The listing builds one solid part. Answer for the finished solid, in the listing's coordinates (mm). A direction names the side the tool comes from. Give positions to 0.01 mm unless a question says otherwise; leave off trailing zeros. Order: outer loops, then holes, each group sorted by start corner. A loop starts at its lowest first (then second) coordinate and runs counter-clockwise, first axis right, second up. Notation, with made-up numbers: (43, 26) - (60, 26) arc R16 ccw to (60, 30) - close; hole circle Ø2 at (85.25, -35). An arc over 180 degrees is marked (long way). Answer as CSV lines item,"result". Start each with the question number.
1. Section C-C on z = 1.9 is taken. Give the vertices of the cut face in (x, y), and give its area (3 significant figures).
2. Section B-B on y = -45 is taken. Give the vertices of the cut face in (x, z), and give its area (4 significant figures).
3. Section D-D on y = -35 is taken. Give the vertices of the cut face in (x, z), and give its area (3 significant figures).
4. Which of the six approach directions +Z, -Z, +X, -X, +Y, -Y give full straight-line access (tool end or side, diameter ignored) to faces 4 (the flat face through (4, -25, 1)), 5 (the flat face through (68, -32, 2.5))?
5. Section A-A on x = 119 is taken. Give the vertices of the cut face in (y, z).
6. A flat-ended cylindrical pin translates along its axis: pin 1 (1.2 mm diameter, centred on x = 132.5, z = 1, fed in from +Y). Find the tip coordinate at first contact, or state that the pin passes through.
7. Determine the mould class of faces 1 (the flat face through (68, -32, 0)), 2 (the flat face through (0, -33, 1)), 3 (the cylindrical face through (117.45, -34.93, 1.27)) for opening direction X: +X half, -X half, draft (parallel to the pull), parting line (faces both ways), or undercut.
8. Consider line 1 along Y through (x, z) = (119, 1.5); line 2 along X through (y, z) = (-6, 2.25); line 3 along X through (y, z) = (-21, 0.7). Determine where each line is inside the solid, lowest interval first. Write a range as [from, to].
from build123d import *

# Parameters (mm, degrees)
CROQUIS1_W              = 138
CROQUIS1_H              = 65
SALIENTE_EXTRUIR1_DEPTH = 2.5
CROQUIS2_W              = 2.5
CROQUIS2_H              = 50
CORTAR_EXTRUIR1_DEPTH   = 2.5
CROQUIS3_R              = 1.55
CORTAR_EXTRUIR2_DEPTH   = 153.562282364


with BuildPart() as part:
    # Croquis1 → Saliente-Extruir1 (new body)
    with BuildSketch(Plane.XY):
        with Locations((69, -32.5)):
            Rectangle(CROQUIS1_W, CROQUIS1_H)
    extrude(amount=SALIENTE_EXTRUIR1_DEPTH)

    # Croquis2 → Cortar-Extruir1 (cut)
    with BuildSketch(Plane.XY.offset(2.5)):
        with Locations((5.25, -25)):
            Rectangle(CROQUIS2_W, CROQUIS2_H)
        with Locations((132.75, -24.997545264)):
            Rectangle(CROQUIS2_W, CROQUIS2_H)
    extrude(amount=-CORTAR_EXTRUIR1_DEPTH, mode=Mode.SUBTRACT)

    # Croquis3 → Cortar-Extruir2 (cut, through all)
    with BuildSketch(Plane.XY.offset(2.5)):
        with Locations((119, -35)):
            Circle(CROQUIS3_R)
        with Locations((119, -20)):
            Circle(CROQUIS3_R)
        with Locations((99, -35)):
            Circle(CROQUIS3_R)
        with Locations((99, -20)):
            Circle(CROQUIS3_R)
        with Locations((79, -35)):
            Circle(CROQUIS3_R)
        with Locations((79, -20)):
            Circle(CROQUIS3_R)
    extrude(amount=-CORTAR_EXTRUIR2_DEPTH, mode=Mode.SUBTRACT)


solid = part.part
Checks:
1,outline,"(0, -65) - (138, -65) - (138, 0) - (134, 0) - (134, -50) - (131.5, -50) - (131.5, 0) - (6.5, 0) - (6.5, -50) - (4, -50) - (4, 0) - (0, 0) - close; hole circle Ø3.1 at (79, -35); hole circle Ø3.1 at (79, -20); hole circle Ø3.1 at (99, -35); hole circle Ø3.1 at (99, -20); hole circle Ø3.1 at (119, -35); hole circle Ø3.1 at (119, -20)"
1,area,"8,670 mm²"
2,outline,"(0, 0) - (4, 0) - (4, 2.5) - (0, 2.5) - close; (6.5, 0) - (131.5, 0) - (131.5, 2.5) - (6.5, 2.5) - close; (134, 0) - (138, 0) - (138, 2.5) - (134, 2.5) - close"
2,area,"332.5 mm²"
3,outline,"(0, 0) - (4, 0) - (4, 2.5) - (0, 2.5) - close; (6.5, 0) - (77.45, 0) - (77.45, 2.5) - (6.5, 2.5) - close; (80.55, 0) - (97.45, 0) - (97.45, 2.5) - (80.55, 2.5) - close; (100.55, 0) - (117.45, 0) - (117.45, 2.5) - (100.55, 2.5) - close; (120.55, 0) - (131.5, 0) - (131.5, 2.5) - (120.55, 2.5) - close; (134, 0) - (138, 0) - (138, 2.5) - (134, 2.5) - close"
3,area,"309 mm²"
4,face 4,"+Z, -Z, +Y"
4,face 5,"+Z, +X, -X, +Y, -Y"
5,outline,"(-65, 0) - (-36.55, 0) - (-36.55, 2.5) - (-65, 2.5) - close; (-33.45, 0) - (-21.55, 0) - (-21.55, 2.5) - (-33.45, 2.5) - close; (-18.45, 0) - (0, 0) - (0, 2.5) - (-18.45, 2.5) - close"
6,pin 1,"stops at y = -50"
7,face 1,"draft"
7,face 2,"-X half"
7,face 3,"undercut"
8,line 1,"y = [-65, -36.55], [-33.45, -21.55], [-18.45, 0]"
8,line 2,"x = [0, 4], [6.5, 131.5], [134, 138]"
8,line 3,"x = [0, 4], [6.5, 77.82], [80.18, 97.82], [100.18, 117.82], [120.18, 131.5], [134, 138]"
